```python
from build123d import *

# Parameters (mm, degrees)
SKIZZE1_W                       = 75
SKIZZE1_H                       = 65
SKIZZE1_W_2                     = 11
SKIZZE1_H_2                     = 20
AUFSATZ_LINEAR_AUSTRAGEN1_DEPTH = 65


with BuildPart() as part:
    # Skizze1 → Aufsatz-Linear austragen1 (new body)
    with BuildSketch(Plane(origin=(0, 0, 0), x_dir=(1, 0, 0), z_dir=(0, 1, 0))):
        Rectangle(SKIZZE1_W, SKIZZE1_H)
        with Locations((-43, -5.5)):
            Rectangle(SKIZZE1_W_2, SKIZZE1_H_2)
        Polygon((-48.5, -47.5), (-48.5, -15.5), (-48.5, 4.5), (-59.5, 4.5), (-59.5, -100.5), (-48.5, -100.5), align=None)
        Polygon((-37.5, -66.284082461), (-37.5, -47.5), (-48.5, -47.5), (-48.5, -100.5), (-48.5, -117.5), (-37.5, -117.5), align=None)
        Polygon((-27.5, -32.5), (-37.5, -32.5), (-37.5, -47.5), (-37.5, -66.284082461), (-37.5, -117.5), (-27.5, -117.5), align=None)
    extrude(amount=AUFSATZ_LINEAR_AUSTRAGEN1_DEPTH)


solid = part.part
```
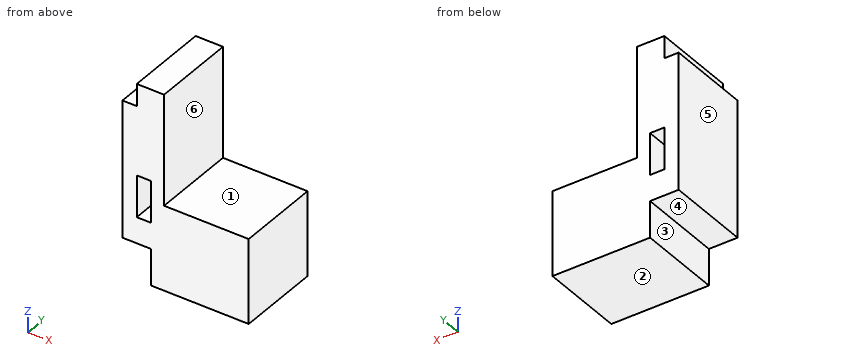
Input: part model. Units: mm. Frame: model coordinates. Face numbers are marked on the shaded views. A direction names the side the tool comes from. Give positions to 0.01 mm unless a question says otherwise; leave off trailing zeros. Order: outer loops, then holes, each group sorted by start corner. A loop starts at its lowest first (then second) coordinate and runs counter-clockwise, first axis right, second up. Notation, with made-up numbers: (48.5, -22) - (65.5, -22) arc R5 cw to (65.5, -14) - close; hole circle Ø8 at (29.5, 56.5). An arc over 180 degrees is marked (long way). Put each result on its own line as item: value.
Item 1: Section query C-C, the plane x = 24.5. Return loops of the section in (y, z), then the cut area to 4 significant figures.
Found:
outline: (0, -32.5) - (65, -32.5) - (65, 32.5) - (0, 32.5) - close
area: 4,225 mm^2
Item 2: Contact query for flat-ended pins moving along their axis: pin 1 (5 mm diameter, centred on y = 29.5, z = 111.5, fed in from -X); pin 2 (6.5 mm diameter, centred on x = -50.5, y = 40.5, fed in from -Z); pin 3 (8.5 mm diameter, centred on y = 23.5, z = -24.5, fed in from -X); pin 4 (12 mm diameter, centred on x = -42, y = 38.5, fed in from -Z). Output: stop coordinate, or through.
Found:
pin 1: stops at x = -48.5
pin 2: stops at z = -4.5
pin 3: stops at x = -37.5
pin 4: stops at z = -32.5
Item 3: Section query D-D, the plane z = -12. Return loops of the section in (x, y).
Found:
outline: (-37.5, 0) - (37.5, 0) - (37.5, 65) - (-37.5, 65) - close
Item 4: Access query for the marked faces 1, 2 and 3. Directions: +Z, -Z, +X, -X, +Y, -Y. A direction counts if a zero-diameter tool reaches every point of the face in a straight line with its end or side. Return the directions, or none.
Found:
face 1: +Z, +X, +Y, -Y
face 2: -Z, +X, -X, +Y, -Y
face 3: -Z, -X, +Y, -Y
Item 5: Section query B-B, the plane y = 14.5. Return loops of the section in (x, z).
Found:
outline: (-59.5, -4.5) - (-37.5, -4.5) - (-37.5, -32.5) - (37.5, -32.5) - (37.5, 32.5) - (-27.5, 32.5) - (-27.5, 117.5) - (-48.5, 117.5) - (-48.5, 100.5) - (-59.5, 100.5) - close; hole (-48.5, 15.5) - (-37.5, 15.5) - (-37.5, 47.5) - (-48.5, 47.5) - close
Item 6: Ray query, L1, parallel to X at y = 51, z = 33; L2, parallel to Z at x = -45.5, y = 41.5; L3, parallel to X at y = 48.5, z = 73.5. Return the intervals inside material, ascending. Write a range as from..to.
Found:
L1: x = -59.5..-48.5, -37.5..-27.5
L2: z = -4.5..15.5, 47.5..117.5
L3: x = -59.5..-27.5
Item 7: Draft query along X for the marked faces 4, 5 and 6. Return one class per face: +X half, -X half, draft (parallel to the pull), parting line (faces both ways), or undercut.
Found:
face 4: draft
face 5: -X half
face 6: +X half
Item 8: Section query A-A, the plane z = 35.5. Return loops of the section in (x, y).
Found:
outline: (-59.5, 0) - (-48.5, 0) - (-48.5, 65) - (-59.5, 65) - close; (-37.5, 0) - (-27.5, 0) - (-27.5, 65) - (-37.5, 65) - close
